```python
from build123d import *
from OCP.BRepFilletAPI import BRepFilletAPI_MakeChamfer

# Parameters (mm, degrees)
SKETCH1_W           = 121
SKETCH1_H           = 110
BOSS_EXTRUDE1_DEPTH = 3
SKETCH8_W           = 3
SKETCH8_H           = 110
BOSS_EXTRUDE5_DEPTH = 3
FILLET4_R           = 2
FILLET5_R           = 5
SKETCH9_W           = 1
SKETCH9_H           = 110
BOSS_EXTRUDE6_DEPTH = 2.5
BOSS_EXTRUDE7_DEPTH = 110
SKETCH11_W          = 24.75
SKETCH11_H          = 107
SKETCH11_W_2        = 49.8
SKETCH11_H_2        = 86.75
CUT_EXTRUDE1_DEPTH  = 3
CHAMFER1_SIZE       = 0.75
CHAMFER1_SIZE2      = 1.299038106
CHAMFER2_SIZE       = 0.75
CHAMFER2_SIZE2      = 1.299038106
SKETCH13_W          = 8
SKETCH13_H          = 22
CUT_EXTRUDE4_DEPTH  = 3
CHAMFER3_SIZE       = 0.75
CHAMFER3_SIZE2      = 1.299038106
CHAMFER4_SIZE       = 1.2
CHAMFER4_SIZE2      = 2.078460969
SKETCH14_W          = 3
SKETCH14_H          = 110
BOSS_EXTRUDE8_DEPTH = 8
SKETCH15_W          = 3.25
SKETCH15_H          = 110
BOSS_EXTRUDE9_DEPTH = 3.5
FILLET6_R           = 2
FILLET7_R           = 5
CUT_EXTRUDE5_START  = -6.5
SKETCH17_W          = 5.25
SKETCH17_H          = 90
CUT_EXTRUDE5_DEPTH  = 6.5
SKETCH18_W          = 3
SKETCH18_H          = 5.101072491
CUT_EXTRUDE6_DEPTH  = 110


with BuildPart() as part:
    # Sketch1 → Boss-Extrude1 (new body)
    with BuildSketch(Plane.XY):
        Rectangle(SKETCH1_W, SKETCH1_H)
    extrude(amount=BOSS_EXTRUDE1_DEPTH)

    # Sketch8 → Boss-Extrude5 (add)
    with BuildSketch(Plane(origin=(0, 0, 0), x_dir=(-1, 0, 0), z_dir=(0, 0, -1))):
        with Locations((-59, 0)):
            Rectangle(SKETCH8_W, SKETCH8_H)
    extrude(amount=BOSS_EXTRUDE5_DEPTH)

    # Fillet4
    fillet4_edges = [part.edges().sort_by_distance(p)[0] for p in [
        (57.5, 0, 0),
    ]]
    fillet(fillet4_edges, radius=FILLET4_R)

    # Fillet5
    fillet5_edges = [part.edges().sort_by_distance(p)[0] for p in [
        (60.5, 0, 3),
    ]]
    fillet(fillet5_edges, radius=FILLET5_R)

    # Sketch9 → Boss-Extrude6 (add)
    with BuildSketch(Plane(origin=(0, 0, -3), x_dir=(-1, 0, 0), z_dir=(0, 0, -1))):
        with Locations((-59, 0)):
            Rectangle(SKETCH9_W, SKETCH9_H)
    extrude(amount=BOSS_EXTRUDE6_DEPTH)

    # Sketch10 → Boss-Extrude7 (add, through all)
    with BuildSketch(Plane(origin=(0, 55, 0), x_dir=(1, 0, 0), z_dir=(0, 1, 0))):
        Polygon((58.5, 5.5), (58, 3), (58.5, 3), align=None)
    extrude(amount=-BOSS_EXTRUDE7_DEPTH)

    # Sketch11 → Cut-Extrude1 (cut)
    with BuildSketch(Plane.XY.offset(3)):
        with Locations((-21.125, 1.5)):
            Rectangle(SKETCH11_W, SKETCH11_H)
        with Locations((29.4, 11.625)):
            Rectangle(SKETCH11_W_2, SKETCH11_H_2)
    extrude(amount=-CUT_EXTRUDE1_DEPTH, mode=Mode.SUBTRACT)

    # Chamfer1
    chamfer1_edges = [part.edges().sort_by_distance(p)[0] for p in [
        (-33.5, 1.5, 3),
        (-21.125, -52, 3),
        (-8.75, 1.5, 3),
    ]]
    chamfer1_side = [part.faces().sort_by_distance(p)[0] for p in [
        (-58.901375591, 0, 3),
    ]]
    chamfer(chamfer1_edges, length=CHAMFER1_SIZE, length2=CHAMFER1_SIZE2, reference=chamfer1_side[0])

    # Chamfer2
    chamfer2_edges = [part.edges().sort_by_distance(p)[0] for p in [
        (-21.125, -52, 0),
    ]]
    chamfer2_side = [part.faces().sort_by_distance(p)[0] for p in [
        (55.340137559, 0, 0),
    ]]
    chamfer(chamfer2_edges, length=CHAMFER2_SIZE, length2=CHAMFER2_SIZE2, reference=chamfer2_side[0])

    # Sketch13 → Cut-Extrude4 (cut)
    with BuildSketch(Plane.XY.offset(3)):
        with Locations((0.5, -9.5)):
            Rectangle(SKETCH13_W, SKETCH13_H)
    extrude(amount=-CUT_EXTRUDE4_DEPTH, mode=Mode.SUBTRACT)

    # Chamfer3: one chamfer whose edges measure the first distance from different faces: ONE call of the kernel's chamfer builder (chamfer() names one face for all edges)
    chamfer3_edges_1 = [part.edges().sort_by_distance(p)[0] for p in [
        (4.5, -26.125, 3),
        (0.5, -20.5, 3),
        (29.4, -31.75, 3),
    ]]
    chamfer3_side_1 = [part.faces().sort_by_distance(p)[0] for p in [
        (-6.401375591, 1.125, 3),
    ]]
    chamfer3_edges_2 = [part.edges().sort_by_distance(p)[0] for p in [
        (0.5, 1.5, 3),
    ]]
    chamfer3_side_2 = [part.faces().sort_by_distance(p)[0] for p in [
        (0.5, 1.5, 1.5),
    ]]
    chamfer3_edges_3 = [part.edges().sort_by_distance(p)[0] for p in [
        (4.5, 28.25, 3),
    ]]
    chamfer3_side_3 = [part.faces().sort_by_distance(p)[0] for p in [
        (4.5, 28.25, 1.5),
    ]]
    chamfer3 = BRepFilletAPI_MakeChamfer(part.part.solid().wrapped)
    for e in chamfer3_edges_1:
        chamfer3.Add(CHAMFER3_SIZE, CHAMFER3_SIZE2, e.wrapped, chamfer3_side_1[0].wrapped)  # the first distance lies on this face
    for e in chamfer3_edges_2:
        chamfer3.Add(CHAMFER3_SIZE, CHAMFER3_SIZE2, e.wrapped, chamfer3_side_2[0].wrapped)  # the first distance lies on this face
    for e in chamfer3_edges_3:
        chamfer3.Add(CHAMFER3_SIZE, CHAMFER3_SIZE2, e.wrapped, chamfer3_side_3[0].wrapped)  # the first distance lies on this face
    add(Compound.cast(chamfer3.Shape()), mode=Mode.REPLACE)

    # Chamfer4
    chamfer4_edges = [part.edges().sort_by_distance(p)[0] for p in [
        (-3.5, -9.225480947, 3),
    ]]
    chamfer4_side = [part.faces().sort_by_distance(p)[0] for p in [
        (-2.399519053, 53.401375591, 3),
    ]]
    chamfer(chamfer4_edges, length=CHAMFER4_SIZE, length2=CHAMFER4_SIZE2, reference=chamfer4_side[0])

    # Sketch14 → Boss-Extrude8 (add)
    with BuildSketch(Plane.ZY.offset(60.5)):
        with Locations((1.5, 0)):
            Rectangle(SKETCH14_W, SKETCH14_H)
    extrude(amount=BOSS_EXTRUDE8_DEPTH)

    # Sketch15 → Boss-Extrude9 (add)
    with BuildSketch(Plane(origin=(0, 0, 0), x_dir=(-1, 0, 0), z_dir=(0, 0, -1))):
        with Locations((66.875, 0)):
            Rectangle(SKETCH15_W, SKETCH15_H)
    extrude(amount=BOSS_EXTRUDE9_DEPTH)

    # Fillet6
    fillet6_edges = [part.edges().sort_by_distance(p)[0] for p in [
        (-65.25, 0, 0),
    ]]
    fillet(fillet6_edges, radius=FILLET6_R)

    # Fillet7
    fillet7_edges = [part.edges().sort_by_distance(p)[0] for p in [
        (-68.5, 0, 3),
    ]]
    fillet(fillet7_edges, radius=FILLET7_R)

    # Sketch17 → Cut-Extrude5 (cut)
    with BuildSketch(Plane(origin=(0, 0, -3.5), x_dir=(-1, 0, 0), z_dir=(0, 0, -1)).offset(CUT_EXTRUDE5_START)):
        with Locations((65.875, -10)):
            Rectangle(SKETCH17_W, SKETCH17_H)
    extrude(amount=CUT_EXTRUDE5_DEPTH, mode=Mode.SUBTRACT)

    # Sketch18 → Cut-Extrude6 (cut)
    with BuildSketch(Plane(origin=(0, 55, 0), x_dir=(1, 0, 0), z_dir=(0, 1, 0))):
        with Locations((59, 5.550536246)):
            Rectangle(SKETCH18_W, SKETCH18_H)
    extrude(amount=-CUT_EXTRUDE6_DEPTH, mode=Mode.SUBTRACT)


solid = part.part
```
The listing builds one solid part. Answer for the finished solid, in the listing's coordinates (mm). A direction names the side the tool comes from. Coordinates: 2 decimals unless noted, no trailing zeros. Loops run counter-clockwise (first coordinate to the right, second up) from the corner with the lowest first, then second, coordinate; pieces in that order, holes last. Notation, with made-up numbers: M 67.25,-35 L 80.25,-35 A13 cw 80.25,-24 Z; hole C 19,7 d4. An arc over 180 degrees is marked long. Answer as a JSON object with one key per item and string values. Group by question number.
Item 1: Section C-C (y = 40.5) is taken. Write down the section's boundary in (x, z).
Item 2: Determine the mould class of faces 5 (the face through (-3, -25, 3)), 6 (the face through (-63.25, -11, 2)), 7 (the face through (54.3, 11, 2)) for opening direction X: +X half, -X half, draft (parallel to the pull), parting line (faces both ways), or undercut.
Item 3: Section B-B (x = 1) is taken. Write down the section's boundary in (y, z), and give its area (3 significant figures).
Item 4: Which of the six approach directions +Z, -Z, +X, -X, +Y, -Y give full straight-line access (tool end or side, diameter ignored) to faces 1 (the face through (59, 1, -3)), 2 (the face through (-67.07, 45.14, 1.5)), 3 (the face through (-66, 35, 0)), 4 (the face through (-3, -25, 0))?
Item 5: Consider L1, parallel to X at y = 28, z = 2; L2, parallel to X at y = -8.5, z = 0.5; L3, parallel to Y at x = 3, z = 0.5. Determine where each line is inside the solid, lowest interval first.
Item 6: Section A-A (y = -6) is taken. Write down the section's boundary in (x, z), and give its area (3 significant figures).
Item 7: Each of these flat-tipped pins is pushed along its axis until it touches: P1, Ø2.5, axis at y = -17, z = 1.5, coming from the -X side; P2, Ø1.9, axis at x = 38, z = 1, coming from the +Y side; P3, Ø1.4, axis at y = -22, z = 1, coming from the +X side; P4, Ø1, axis at x = -45, z = -1, coming from the +Y side. Where does it stop, or does it pass through?
Item 8: Section D-D (x = 15.5) is taken. Write down the section's boundary in (y, z).
Solved:
{
 "1": {"outline": "M -68.5,-3.5 L -65.25,-3.5 L -65.25,-2 A2 cw -63.25,0 L -33.5,0 L -33.5,1.7 L -34.25,3 L -63.5,3 A5 ccw -68.5,-2 Z; M -8.75,0 L 4.5,0 L 4.5,2.25 L 3.2,3 L -8,3 L -8.75,1.7 Z; M 54.3,0 L 55.5,0 A2 cw 57.5,-2 L 57.5,-3 L 60.5,-3 L 60.5,-2 A5 ccw 55.5,3 L 54.3,3 Z"},
 "2": {"face 5": "draft", "face 6": "-X half", "face 7": "undercut"},
 "3": {"outline": "M -55,0 L -20.5,0 L -20.5,1.7 L -21.25,3 L -55,3 Z; M 1.5,0 L 55,0 L 55,3 L 2.8,3 L 1.5,2.25 Z", "area": "263 mm2"},
 "4": {"face 1": "-Z, +X, +Y, -Y", "face 2": "+Z, -X, +Y, -Y", "face 3": "+Z, -Z, -X, -Y", "face 4": "-Z, +Y, -Y"},
 "5": {"L1": "x = -63.25 to -33.67, -8.58 to 4.5, 54.3 to 58.5", "L2": "x = -63.25 to -33.5, -8.75 to -3.5, 54.3 to 59.83", "L3": "y = -55 to -20.5, 1.5 to 55"},
 "6": {"outline": "M -63.25,0 L -33.5,0 L -33.5,1.7 L -34.25,3 L -63.25,3 Z; M -8.75,0 L -3.5,0 L -3.5,0.92 L -4.7,3 L -8,3 L -8.75,1.7 Z; M 54.3,0 L 55.5,0 A2 cw 57.5,-2 L 57.5,-3 L 60.5,-3 L 60.5,-2 A5 ccw 55.5,3 L 54.3,3 Z", "area": "126 mm2"},
 "7": {"P1": "stops at x = -63.25", "P2": "stops at y = -31.75", "P3": "stops at x = 59.94", "P4": "passes through"},
 "8": {"outline": "M -55,0 L -31.75,0 L -31.75,1.7 L -32.5,3 L -55,3 Z"}
}
